Check sheet for the modelled part. Datum: model origin and axes. Units: mm. A direction names the side the tool comes from. Give positions to 0.01 mm unless a question says otherwise; leave off trailing zeros. Loops run counter-clockwise (first coordinate to the right, second up) from the corner with the lowest first, then second, coordinate; pieces in that order, holes last. Notation, with made-up numbers: (-4.5, -13) -> (15.5, -13) arc R13 cw to (15.5, 11) -> close; hole circle Ø1 at (32.5, -31.5). An arc over 180 degrees is marked (long way). Write each question's results on one line, items separated by ' | '. Start each with the question number.
1. Cross-section at A-A on z = 14.25. Record the boundary of the cut face in (x, y) (1 decimal).
2. Tool access check on faces 1 (the face through (-0.964, -9.515, 20.928)), 2 (the face through (-16.02, -5.91, 18.39)), 3 (the face through (25.4, 0, 9)). Record the directions out of +Z, -Z, +X, -X, +Y, -Y that give a thin tool (end or side, any length) a straight path to the whole face; none if there is none.
3. Cross-section at D-D on y = 8. Record the boundary of the cut face in (x, z), and give its area (3 significant figures).
4. Gauge pin test, flat ends, axial feed: pin 1 Ø9 at (x, y) = (-9.525, 0) entering from -Z; pin 2 Ø1.1 at (x, y) = (-0.5, -4.5) entering from -Z; pin 3 Ø2 at (x, y) = (9.5, 1.5) entering from -Z. Record the tip position at first contact, or that the pin passes through.
5. Cross-section at B-B on x = -17.78. Record the boundary of the cut face in (y, z), and give its area (3 significant figures).
6. Cross-section at C-C on y = 0. Record the boundary of the cut face in (x, z).
7. Mould release check, pull along Y, two halves, no side actions. Record for faces 4 (the face through (-0.413, 3.316, 18.388)), 5 (the face through (0, 5, 22.86)): +Y half, -Y half, draft (parallel to the pull), parting line (faces both ways), or undercut.
8. Material ranges on L1, parallel to X at y = 0, z = 4; L2, parallel to Y at x = 0, z = 17.8; L3, parallel to Y at x = 20, z = 12, recorded low to high. Write a range as from..to.
from build123d import *

# Parameters (mm, degrees)
F0_W     = 50.8
F0_H     = 25.4
F1_DEPTH = 19.05
F2_R     = 4.445
F3_DEPTH = 3.81
F4_T     = -2.54
F5_R     = 5.9055
F5_R_2   = 3.3655
F6_DEPTH = 16.51


with BuildPart() as f1:
    # F0 (on Top) → F1 (new body)
    with BuildSketch(Plane.XY):
        Rectangle(F0_W, F0_H)
    extrude(amount=F1_DEPTH)

    # F2 (on face) → F3 (join)
    with BuildSketch(Plane.XY.offset(19.05)):
        with Locations((-17.78, 5.1759317036)):
            Circle(F2_R)
        with Locations((0, 5.1759317036)):
            Circle(F2_R)
        with Locations((17.78, 5.1759317036)):
            Circle(F2_R)
        with Locations((17.78, -5.1759317036)):
            Circle(F2_R)
        with Locations((0, -5.1759317036)):
            Circle(F2_R)
        with Locations((-17.78, -5.1759317036)):
            Circle(F2_R)
    extrude(amount=F3_DEPTH)

    # F4
    f4_openings = [f1.faces().sort_by_distance(p)[0] for p in [
        (0, 0, 0),
    ]]
    offset(amount=F4_T, openings=f4_openings, kind=Kind.INTERSECTION)

    # F5 (on face) → F6 (join, through all)
    with BuildSketch(Plane(origin=(0, 0, 0), x_dir=(1, 0, 0), z_dir=(0, 0, -1))):
        with Locations((-9.525, 0)):
            Circle(F5_R)
        with Locations((-9.525, 0)):
            Circle(F5_R_2, mode=Mode.SUBTRACT)
        with Locations((9.525, 0)):
            Circle(F5_R)
        with Locations((9.525, 0)):
            Circle(F5_R_2, mode=Mode.SUBTRACT)
    extrude(amount=-F6_DEPTH)


solid = f1.part
Geometry says:
1) outline: (-25.4, -12.7) -> (25.4, -12.7) -> (25.4, 12.7) -> (-25.4, 12.7) -> close; circle Ø11.8 at (-9.5, 0); circle Ø11.8 at (9.5, 0); hole (-22.9, -10.2) -> (22.9, -10.2) -> (22.9, 10.2) -> (-22.9, 10.2) -> close; hole circle Ø6.7 at (-9.5, 0); hole circle Ø6.7 at (9.5, 0)
2) face 1: +Z | face 2: -Z | face 3: +Z, -Z, +X, +Y, -Y
3) outline: (-25.4, 0) -> (-22.86, 0) -> (-22.86, 16.51) -> (22.86, 16.51) -> (22.86, 0) -> (25.4, 0) -> (25.4, 19.05) -> (21.21, 19.05) -> (21.21, 22.86) -> (14.35, 22.86) -> (14.35, 19.05) -> (3.43, 19.05) -> (3.43, 22.86) -> (-3.43, 22.86) -> (-3.43, 19.05) -> (-14.35, 19.05) -> (-14.35, 22.86) -> (-21.21, 22.86) -> (-21.21, 19.05) -> (-25.4, 19.05) -> close | area: 291 mm^2
4) pin 1: z = 0 | pin 2: z = 20.32 | pin 3: z = 16.51
5) outline: (-12.7, 0) -> (-10.16, 0) -> (-10.16, 16.51) -> (-7.08, 16.51) -> (-7.08, 20.32) -> (-3.27, 20.32) -> (-3.27, 16.51) -> (3.27, 16.51) -> (3.27, 20.32) -> (7.08, 20.32) -> (7.08, 16.51) -> (10.16, 16.51) -> (10.16, 0) -> (12.7, 0) -> (12.7, 19.05) -> (9.62, 19.05) -> (9.62, 22.86) -> (0.73, 22.86) -> (0.73, 19.05) -> (-0.73, 19.05) -> (-0.73, 22.86) -> (-9.62, 22.86) -> (-9.62, 19.05) -> (-12.7, 19.05) -> close | area: 187 mm^2
6) outline: (-25.4, 0) -> (-22.86, 0) -> (-22.86, 16.51) -> (-15.43, 16.51) -> (-15.43, 0) -> (-12.89, 0) -> (-12.89, 16.51) -> (-6.16, 16.51) -> (-6.16, 0) -> (-3.62, 0) -> (-3.62, 16.51) -> (3.62, 16.51) -> (3.62, 0) -> (6.16, 0) -> (6.16, 16.51) -> (12.89, 16.51) -> (12.89, 0) -> (15.43, 0) -> (15.43, 16.51) -> (22.86, 16.51) -> (22.86, 0) -> (25.4, 0) -> (25.4, 19.05) -> (-25.4, 19.05) -> close
7) face 4: undercut | face 5: draft
8) L1: -25.4..-22.86, -15.43..-12.89, -6.16..-3.62, 3.62..6.16, 12.89..15.43, 22.86..25.4 | L2: -12.7..-7.08, -3.27..3.27, 7.08..12.7 | L3: -12.7..-10.16, 10.16..12.7
